Part model, mm, in its own coordinate system. Face numbers are marked on the shaded views. A direction names the side the tool comes from. Give positions to 0.01 mm unless a question says otherwise; leave off trailing zeros. Order: outer loops, then holes, each group sorted by start corner. A loop starts at its lowest first (then second) coordinate and runs counter-clockwise, first axis right, second up. Notation, with made-up numbers: (7, 67.25) - (25, 67.25) arc R29 cw to (25, 102.25) - close; hole circle Ø4 at (-21, 59). An arc over 180 degrees is marked (long way). One line per item, written item: value.
```python
from build123d import *

# Parameters (mm, degrees)
BOSS_EXTRUDE1_DEPTH                               = 3.048
BOSS_EXTRUDE2_DEPTH                               = 29.971999999999998
BOSS_EXTRUDE3_DEPTH                               = 3.048
BOSS_EXTRUDE4_DEPTH                               = 3.048
SKETCH13_W                                        = 29.972
SKETCH13_H                                        = 48.7
BOSS_EXTRUDE5_DEPTH                               = 3.048
CSK_FOR_4_FLAT_HEAD_MACHINE_SCREW_100_D           = 2.9464
CSK_FOR_4_FLAT_HEAD_MACHINE_SCREW_100_CSINK_D     = 5.715
CSK_FOR_4_FLAT_HEAD_MACHINE_SCREW_100_CSINK_ANGLE = 100
CUT_EXTRUDE1_DEPTH                                = 1.397
CUT_EXTRUDE1_DEPTH_BACK                           = 1.397
SKETCH15_R                                        = 9.184035329670005
SKETCH15_R_2                                      = 8.124741076595411
SKETCH15_R_3                                      = 8.201451240556812
SKETCH15_R_4                                      = 5.810172256980604
BOSS_EXTRUDE6_DEPTH                               = 3.048
CSK_FOR_4_FLAT_HEAD_MACHINE_SCREW1_AT_2_COUNT     = 2
CSK_FOR_4_FLAT_HEAD_MACHINE_SCREW1_AT_2_PITCH     = 35.474094707842795
CSK_FOR_4_FLAT_HEAD_MACHINE_SCREW1_AT_3_COUNT     = 2
CSK_FOR_4_FLAT_HEAD_MACHINE_SCREW1_AT_3_PITCH     = 43.70753982500484
CSK_FOR_4_FLAT_HEAD_MACHINE_SCREW1_AT_4_COUNT     = 2
CSK_FOR_4_FLAT_HEAD_MACHINE_SCREW1_AT_4_PITCH     = 25.069264350610375
CUT_EXTRUDE2_DEPTH                                = 3.048
FILLET3_R                                         = 3.8099999999999996
FILLET4_R                                         = 1.27
SKETCH21_W                                        = 2.540000000000001
SKETCH21_H                                        = 33.02
CUT_EXTRUDE3_DEPTH                                = 77.47
FILLET5_R                                         = 0.508
FILLET6_R                                         = 0.508
SKETCH22_W                                        = 123.04970813102194
SKETCH22_H                                        = 134.7131875745612
CUT_EXTRUDE4_DEPTH                                = 77.47


with BuildPart() as part:
    # Sketch2 → Boss-Extrude1 (new body)
    with BuildSketch(Plane.XY):
        Polygon((-47.58059551455695, 48.12489153745831), (-22.21147896413696, 6.554494312375088), (5.701292889255674, 23.58878817682547), (-19.667823661164306, 65.1591854019087), align=None)
        Polygon((-38.85234269167306, 46.0124042215628), (-20.098991648241444, 15.282747135258976), (-3.0269599336282123, 25.701275492720985), (-21.78031097705982, 56.430932579024805), align=None, mode=Mode.SUBTRACT)
    extrude(amount=BOSS_EXTRUDE1_DEPTH)

    # Sketch3 → Boss-Extrude2 (add)
    with BuildSketch(Plane.XY.offset(3.048)):
        Polygon((2.4490708476218597, 21.604058524728963), (-22.920045702798127, 63.17445574981219), (-44.328373472923126, 50.10962118955482), (-18.95925692250314, 8.539223964471608), align=None)
        Polygon((-38.85234269167306, 46.0124042215628), (-20.098991648241444, 15.282747135258976), (-3.0269599336282087, 25.701275492720985), (-21.78031097705982, 56.430932579024805), align=None, mode=Mode.SUBTRACT)
    extrude(amount=BOSS_EXTRUDE2_DEPTH)

    # Sketch4 → Boss-Extrude3 (add)
    with BuildSketch(Plane.XY.offset(33.02)):
        Polygon((-38.85234269167306, 46.0124042215628), (-37.46131723814535, 43.733039051773666), (-20.389285523532113, 54.15156740923567), (-21.78031097705982, 56.430932579024805), align=None)
        Polygon((-29.47566716995725, 30.647575678410885), (-12.403635455344016, 41.0661040358729), (-3.0269599336282087, 25.701275492720985), (-20.098991648241444, 15.282747135258976), align=None)
    extrude(amount=-BOSS_EXTRUDE3_DEPTH)

    # Sketch12 → Boss-Extrude4 (add)
    with BuildSketch(Plane.XY.offset(3.048)):
        Polygon((2.4490708476218597, 21.604058524728963), (5.701292889255674, 23.58878817682547), (8.120429940678708, 25.065112049236276), (-17.248686609741274, 66.6355092743195), (-22.920045702798127, 63.17445574981219), align=None)
    extrude(amount=-BOSS_EXTRUDE4_DEPTH)

    # Sketch13 → Boss-Extrude5 (add)
    with BuildSketch(Plane(origin=(11.391019162328917, 6.95158362794815, 0), x_dir=(0, 0, -1), z_dir=(0.8536015857306615, 0.5209264178731006, 0))):
        with Locations((-18.034000000000002, 41.515472911157566)):
            Rectangle(SKETCH13_W, SKETCH13_H)
    extrude(amount=BOSS_EXTRUDE5_DEPTH)

    # CSK for #4 Flat Head Machine Screw (100)2 (through all)
    with Locations(Plane(origin=(-10.017308607796087, -6.113250932309213, 0), x_dir=(0, 0, 1), z_dir=(-0.8536015857306615, -0.5209264178731007, 0))):
        with Locations((27.397617355, 61.471448289), (7.925915452, 61.471448289), (7.925915452, 21.515515982), (27.397617355, 21.515515982)):
            CounterSinkHole(CSK_FOR_4_FLAT_HEAD_MACHINE_SCREW_100_D / 2, CSK_FOR_4_FLAT_HEAD_MACHINE_SCREW_100_CSINK_D / 2, counter_sink_angle=CSK_FOR_4_FLAT_HEAD_MACHINE_SCREW_100_CSINK_ANGLE)

    # Sketch14 → Cut-Extrude1 (cut, two sides: drawn at the far end of the back side and taken through both)
    with BuildSketch(Plane(origin=(11.607833965104508, 7.083898938087922, 0), x_dir=(0, 0, -1), z_dir=(0.8536015857306615, 0.5209264178731005, 0)).offset(-CUT_EXTRUDE1_DEPTH_BACK)):
        Polygon((-30.697174143874744, 19.61051598216394), (-30.697174143874744, 14.979833054183299), (-24.09806056703731, 14.979833054183299), (-24.09806056703731, 19.610515982163985), (-24.098060567037347, 23.42051598216399), (-27.39761735545604, 25.325515982163957), (-30.697174143874758, 23.420515982163952), align=None)
        Polygon((-27.39761735545604, 57.661448288693826), (-24.098060567037333, 59.56644828869383), (-24.098060567037336, 63.37644828869381), (-24.098060567037336, 70.99644828869384), (-30.69717414387474, 70.99644828869384), (-30.69717414387474, 63.37644828869381), (-30.69717414387474, 59.56644828869381), align=None)
        Polygon((-7.925915451689084, 57.661448288693826), (-4.626358663270381, 59.56644828869382), (-4.626358663270402, 63.37644828869381), (-4.626358663270402, 70.99644828869384), (-11.225472240107786, 70.99644828869384), (-11.225472240107786, 63.376448288693766), (-11.225472240107747, 59.566448288693785), align=None)
        Polygon((-7.925915451689081, 25.325515982163946), (-11.225472240107791, 23.42051598216395), (-11.225472240107791, 19.610515982163946), (-11.225472240107791, 14.979833054183299), (-4.626358663270366, 14.979833054183299), (-4.626358663270366, 19.610515982163953), (-4.6263586632703655, 23.420515982163952), align=None)
    extrude(amount=CUT_EXTRUDE1_DEPTH + CUT_EXTRUDE1_DEPTH_BACK, mode=Mode.SUBTRACT)

    # Sketch15 → Boss-Extrude6 (add)
    with BuildSketch(Plane(origin=(0, 0, 0), x_dir=(-1, 0, 0), z_dir=(0, 0, -1))):
        with Locations((9.758086495919196, 54.36124573948299)):
            Circle(SKETCH15_R)
        with Locations((39.927818301519274, 35.58488100974543)):
            Circle(SKETCH15_R_2)
        with Locations((25.610425726235285, 18.04643091882164)):
            Circle(SKETCH15_R_3)
        with Locations((-3.4576236647063787, 32.70568986323082)):
            Circle(SKETCH15_R_4)
    extrude(amount=-BOSS_EXTRUDE6_DEPTH)

    # Sketch19 → CSK for #4 Flat Head Machine Screw1 (revolve, cut)
    with BuildSketch(Plane(origin=(3.764373982237945, 32.86032278852424, 3.048), x_dir=(0, -1, 0), z_dir=(1, 0, 0))):
        Polygon((0, 0), (-7.5e-16, 3.0480000000000023), (1.4731999999999932, 3.0480000000000023), (1.4731999999999934, 1.59245498611605), (2.857499999999999, -1.73e-15), align=None)
    csk_for_4_flat_head_machine_screw1 = revolve(axis=Axis((3.764373982237945, 32.86032278852424, 9.39799999999999), (0, 0, -1)), mode=Mode.SUBTRACT)

    # CSK for #4 Flat Head Machine Screw1 at 2: CSK for #4 Flat Head Machine Screw1 ×2
    with Locations(*[Vector(-0.8506492202713736, -0.5257336816789507, 0) * (i * CSK_FOR_4_FLAT_HEAD_MACHINE_SCREW1_AT_2_PITCH) for i in range(1, CSK_FOR_4_FLAT_HEAD_MACHINE_SCREW1_AT_2_COUNT)]):
        add(csk_for_4_flat_head_machine_screw1, mode=Mode.SUBTRACT)

    # CSK for #4 Flat Head Machine Screw1 at 3: CSK for #4 Flat Head Machine Screw1 ×2
    with Locations(*[Vector(-0.997755305773639, 0.06696528802709796, 0) * (i * CSK_FOR_4_FLAT_HEAD_MACHINE_SCREW1_AT_3_PITCH) for i in range(1, CSK_FOR_4_FLAT_HEAD_MACHINE_SCREW1_AT_3_COUNT)]):
        add(csk_for_4_flat_head_machine_screw1, mode=Mode.SUBTRACT)

    # CSK for #4 Flat Head Machine Screw1 at 4: CSK for #4 Flat Head Machine Screw1 ×2
    with Locations(*[Vector(-0.5210117203175807, 0.8535495224600124, 0) * (i * CSK_FOR_4_FLAT_HEAD_MACHINE_SCREW1_AT_4_PITCH) for i in range(1, CSK_FOR_4_FLAT_HEAD_MACHINE_SCREW1_AT_4_COUNT)]):
        add(csk_for_4_flat_head_machine_screw1, mode=Mode.SUBTRACT)

    # Sketch20 → Cut-Extrude2 (cut)
    with BuildSketch(Plane(origin=(0, 0, 0), x_dir=(-1, 0, 0), z_dir=(0, 0, -1))):
        with BuildLine():
            Line((14.542293121824187, 62.20075286029573), (11.563953125478477, 57.32037886408755))
            ThreePointArc((11.563953125478477, 57.32037886408755), (6.044784522535942, 56.24291105550805), (7.610320649443919, 50.84186897257834))
            Line((7.610320649443919, 50.84186897257834), (-1.4954062126549716, 35.92102291440944))
            ThreePointArc((-1.4954062126549716, 35.92102291440944), (-7.016596023871767, 34.845052440620755), (-5.448804035753348, 29.442897530407524))
            Line((-5.448804035753348, 29.442897530407524), (-6.484295885760952, 27.746117611303884))
            Line((-6.484295885760952, 27.746117611303884), (-6.762670750549963, 27.28996638176623))
            Line((-6.762670750549963, 27.28996638176623), (-14.061950278269341, 31.74448896114331))
            Line((-14.061950278269341, 31.74448896114331), (8.559037851416688, 68.81174198534737))
            Line((8.559037851416688, 68.81174198534737), (14.542293121824187, 65.16034795406075))
            Line((14.542293121824187, 65.16034795406075), (14.542293121824187, 62.20075286029573))
        make_face()
        Polygon((21.78031097705982, 56.430932579024805), (38.85234269167306, 46.0124042215628), (20.098991648241444, 15.282747135258976), (3.0269599336282123, 25.701275492720985), align=None)
        with BuildLine():
            Line((22.21147896413696, 6.554494312375088), (24.781951964671258, 10.766528400207497))
            ThreePointArc((24.781951964671258, 10.766528400207497), (29.66385906245521, 12.225666721445755), (28.72915433514684, 17.23450177808784))
            Line((28.72915433514684, 17.23450177808784), (38.012718373529104, 32.44675577885475))
            ThreePointArc((38.012718373529104, 32.44675577885475), (43.097277822107074, 33.802481129765034), (41.97793801322115, 38.944252653808825))
            Line((41.97793801322115, 38.944252653808825), (47.58059551455695, 48.12489153745831))
            Line((47.58059551455695, 48.12489153745831), (51.80171473929435, 35.787210781861546))
            Line((51.80171473929435, 35.787210781861546), (47.57680035710003, 5.227667032097241))
            Line((47.57680035710003, 5.227667032097241), (22.21147896413696, 6.554494312375088))
        make_face()
    extrude(amount=-CUT_EXTRUDE2_DEPTH, mode=Mode.SUBTRACT)


with BuildPart() as body_2:
    # of the pieces the cut leaves, the one that is kept (cut_extrude2_keep)
    add(part.part.solids().sort_by_distance((-47.580595515, 48.124891537, 0))[0])

    # Fillet3
    fillet3_edges = [body_2.edges().sort_by_distance(p)[0] for p in [
        (-17.248686609741274, 66.6355092743195, 1.524),
        (-47.58059551455695, 48.12489153745831, 1.524),
        (-22.21147896413696, 6.554494312375088, 1.524),
        (8.120429940678708, 25.065112049236276, 1.524),
    ]]
    fillet(fillet3_edges, radius=FILLET3_R)

    # Fillet4
    fillet4_edges = [body_2.edges().sort_by_distance(p)[0] for p in [
        (1.4954062126549714, 35.92102291440944, 1.524),
        (-24.781951964671258, 10.766528400207495, 1.524),
        (-28.72915433514684, 17.23450177808784, 1.524),
        (-38.0127183735291, 32.44675577885475, 1.524),
        (-41.97793801322115, 38.94425265380882, 1.524),
        (-11.563953125478475, 57.320378864087544, 1.524),
        (-7.610320649443917, 50.84186897257834, 1.524),
    ]]
    fillet(fillet4_edges, radius=FILLET4_R)

    # Sketch21 → Cut-Extrude3 (cut)
    with BuildSketch(Plane(origin=(-8.941948314707059, 14.652474896780824, 0), x_dir=(0.8536015857306616, 0.5209264178731006, 0), z_dir=(0.5209264178731005, -0.8536015857306615, 0))):
        with Locations((2.2216732427396275, 16.51)):
            Rectangle(SKETCH21_W, SKETCH21_H)
    extrude(amount=-CUT_EXTRUDE3_DEPTH, mode=Mode.SUBTRACT)


with BuildPart() as cut_extrude3_piece_1:
    # of the separate pieces the step leaves, piece 1, a body of its own (cut_extrude3_pieces)
    add(body_2.part.solids().sort_by_distance((-12.188709065, 58.344117807, 0))[0])

    # Fillet6
    fillet6_edges = [cut_extrude3_piece_1.edges().sort_by_distance(p)[0] for p in [
        (-7.633709794281099, 43.97704085894782, 3.048),
    ]]
    fillet(fillet6_edges, radius=FILLET6_R)


with BuildPart() as cut_extrude3_piece_2:
    # of the separate pieces the step leaves, piece 2, a body of its own (cut_extrude3_pieces)
    add(body_2.part.solids().sort_by_distance((-42.532157132, 39.852408399, 0))[0])

    # Fillet5
    fillet5_edges = [cut_extrude3_piece_2.edges().sort_by_distance(p)[0] for p in [
        (-31.64381519771313, 29.324422577013216, 3.048),
    ]]
    fillet(fillet5_edges, radius=FILLET5_R)

    # Sketch22 → Cut-Extrude4 (cut)
    with BuildSketch(Plane(origin=(2.067982642978631, 1.2620252919381492, 0), x_dir=(0, 0, -1), z_dir=(0.8536015857306616, 0.5209264178731006, 0))):
        with Locations((-42.687564536567926, 74.45417523171726)):
            Rectangle(SKETCH22_W, SKETCH22_H)
    extrude(amount=-CUT_EXTRUDE4_DEPTH, mode=Mode.SUBTRACT)


solid = cut_extrude3_piece_1.part
```
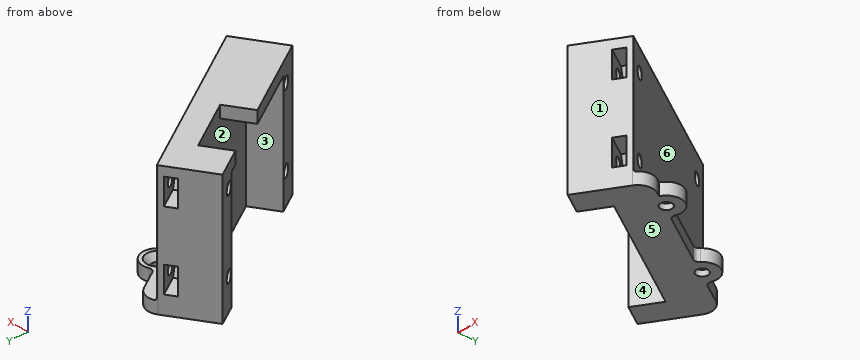
1) Wall check: line 1 along X through (y, z) = (23, 26.5); line 2 along Z through (x, y) = (-25, 56.5); line 3 along Z through (x, y) = (0, 38). Give the ranges that are in metal, low to high. Write a range as [from, to].
Answer:
line 1: x = [-7.45, -5.86], [-1.37, 0.26], [3.53, 4.74]
line 2: z = [0, 6.47], [9.38, 25.94], [28.85, 33.02]
line 3: z = [0, 3.05]
2) Two-plate mould, pull along X, no slides. Class the marked faces 3, 4, 5 and 6: pulls with the +X half, pulls with the -X half, needs draft (parallel to the pull), parting line crosses it, or undercut.
Answer:
face 3: pulls with the -X half
face 4: undercut
face 5: needs draft
face 6: pulls with the +X half
3) Slice it at C-C on z = 31.5. Write the cut outline in (x, y).
Answer:
outline: (-31.33, 58.04) - (-26.63, 50.34) - (-20.39, 54.15) - (-12.4, 41.07) - (-18.65, 37.26) - (-5.96, 16.47) - (4.87, 23.08) arc R3.81 ccw to (5.05, 23.2) - (-20.32, 64.76) arc R3.81 ccw to (-20.5, 64.65) - close
4) Drop flat-ended pins along their axis: P1, Ø8, axis at x = -11, y = 30.5, coming from the -Z side; P2, Ø6, axis at y = 50.5, z = 7.5, coming from the +X side; P3, Ø10, axis at x = -6.5, z = 27, coming from the +Y side; P4, Ø6, axis at x = -5, z = 6.5, coming from the -Y side. Give the stop position or say it passes through.
Answer:
P1: stops at z = 29.97
P2: stops at x = -9.78
P3: stops at y = 50.31
P4: stops at y = 16.47
5) Slice it at B-B on z = 12.5. Write the cut outline in (x, y).
Answer:
outline: (-31.33, 58.04) - (-28.02, 52.62) - (-21.78, 56.43) - (-3.03, 25.7) - (-9.27, 21.89) - (-5.96, 16.47) - (4.87, 23.08) arc R3.81 ccw to (5.05, 23.2) - (-20.32, 64.76) arc R3.81 ccw to (-20.5, 64.65) - close
6) Slice it at A-A on z = 28. Count the separate pieces of the cut face and the enclosed holes in it, then the cut area to 3 significant figures.
Answer:
separate pieces: 5
enclosed holes: 0
area: 267 mm2
7) Which spindle directions (+Z, -Z, +X, -X, +Y, -Y) get a long thin tool onto all of the face, cutting with end or side? Do the marked faces 1 and 2. Say none if no direction does.
Answer:
face 1: +Z, -Z, +X, -Y
face 2: -Z
